Check sheet for the modelled part. Datum: model origin and axes. Units: mm. Face numbers are marked on the shaded views. A direction names the side the tool comes from. Round coordinates to 2 decimals unless told otherwise and drop trailing zeros. Loops run counter-clockwise (first coordinate to the right, second up) from the corner with the lowest first, then second, coordinate; pieces in that order, holes last. Notation, with made-up numbers: (58, 76.5) - (65, 76.5) arc R17 cw to (65, 85.5) - close; hole circle Ø5 at (-31, 81). An arc over 180 degrees is marked (long way). Answer in a Markdown table with one row per item. Add a question column.
(1) Cross-section at B-B on z = 1. Count the separate pieces of the cut face and the enclosed holes in it, then the cut area to 3 significant figures.
(2) Access from +Z, -Z, +X, -X, +Y, -Y to the whole of each face (thin tool, end or side, straight path). Record for the marked faces 5, 6 and 7.
(3) Thickness scan on line 1 along X through (y, z) = (-0.75, 3.25); line 2 along Y through (x, z) = (-17.5, 3.5); line 3 along Y through (x, z) = (-5, 3). Record the ranges inside material, lowest first.
(4) Mould release check, pull along X, two halves, no side actions. Record for the marked faces 1, 2, 3 and 4: +X half, -X half, draft (parallel to the pull), parting line (faces both ways), or undercut.
(5) Cross-section at A-A on x = -26. Enter the section's corners in (y, z).
(6) Gauge pin test, flat end, axial feed: pin 1 (3.5 mm diameter, centred on x = 3, z = 4, fed in from -Y). Record the tip position at first contact, or that the pin passes through.
from build123d import *

# Parameters (mm, degrees)
F0_W     = 20
F0_H     = 3.5
F1_DEPTH = 7
F2_R     = 0.99999
F3_R     = 2


# Not quite as in the source:
# - two fillets or chamfers of one size are made in one step
# - a fillet or chamfer is up to 0.001 mm smaller than in the source, because OpenCascade refuses the exact size


with BuildPart() as f1:
    # F0 (on Top) → F1 (new body)
    with BuildSketch(Plane.XY):
        Polygon((35, -4), (35, 4), (-35, 4), (-35, -4), (-9.7500002012, -4), (-9.7500002012, -2), (9.75, -2), (9.75, -4), align=None)
        with Locations((-22.75, 0)):
            Rectangle(F0_W, F0_H, mode=Mode.SUBTRACT)
        with Locations((22.75, 0)):
            Rectangle(F0_W, F0_H, mode=Mode.SUBTRACT)
    extrude(amount=F1_DEPTH)

    # F2 (radius 1 in the source; OpenCascade refuses exactly that, so slightly less here)
    f2_edges = [f1.edges().sort_by_distance(p)[0] for p in [
        (32.75, 1.75, 3.5),
        (12.75, 1.75, 3.5),
        (12.75, -1.75, 3.5),
        (32.75, -1.75, 3.5),
        (-12.75, -1.75, 3.5),
        (-12.75, 1.75, 3.5),
        (-32.75, 1.75, 3.5),
        (-32.75, -1.75, 3.5),
        (-9.75, -4, 3.5),
        (-9.75, -2, 3.5),
        (9.75, -2, 3.5),
        (9.75, -4, 3.5),
    ]]
    fillet(f2_edges, radius=F2_R)

    # F3
    f3_edges = [f1.edges().sort_by_distance(p)[0] for p in [
        (35, -4, 3.5),
        (35, 4, 3.5),
        (-35, -4, 3.5),
        (-35, 4, 3.5),
    ]]
    fillet(f3_edges, radius=F3_R)


solid = f1.part
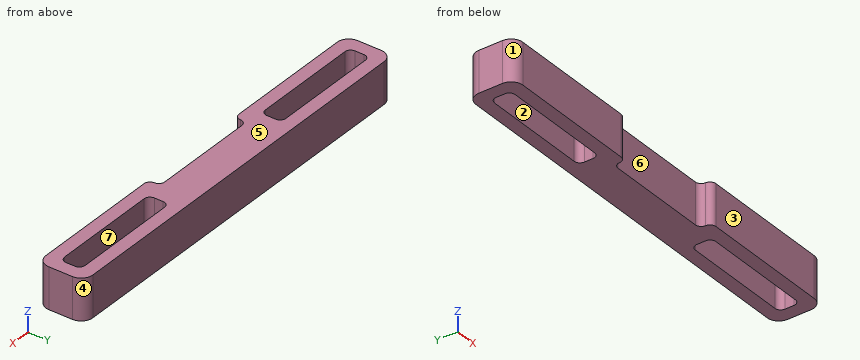
Answers:
| question | item | result |
|---|---|---|
| 1 | separate pieces | 1 |
| 1 | enclosed holes | 2 |
| 1 | area | 379 mm^2 |
| 2 | face 5 | +Z, +X, -X, +Y, -Y |
| 2 | face 6 | +Z, -Z, -Y |
| 2 | face 7 | +Z, -Z |
| 3 | line 1 | x = -35 to -32.75, -12.75 to 12.75, 32.75 to 35 |
| 3 | line 2 | y = -4 to -1.75, 1.75 to 4 |
| 3 | line 3 | y = -2 to 4 |
| 4 | face 1 | -X half |
| 4 | face 2 | undercut |
| 4 | face 3 | draft |
| 4 | face 4 | +X half |
| 5 | outline | (-4, 0) - (-1.75, 0) - (-1.75, 7) - (-4, 7) - close; (1.75, 0) - (4, 0) - (4, 7) - (1.75, 7) - close |
| 6 | pin 1 | stops at y = -2 |
